```python
from build123d import *

# Parameters (mm, degrees)
SKETCH1_W           = 44.45
SKETCH1_H           = 25.4
BOSS_EXTRUDE1_DEPTH = 28.575
SHELL1_T            = -3.175
SKETCH2_W           = 38.1
SKETCH2_H           = 12.7
CUT_EXTRUDE1_DEPTH  = 26.4
CUT_EXTRUDE2_DEPTH  = 45.45
CUT_EXTRUDE3_DEPTH  = 4.175
FILLET1_R           = 6.35
FILLET2_R           = 1.5875
SKETCH6_R           = 9.525
CUT_EXTRUDE4_DEPTH  = 1.905


with BuildPart() as part:
    # Sketch1 → Boss-Extrude1 (new body)
    with BuildSketch(Plane(origin=(0, 0, 0), x_dir=(1, 0, 0), z_dir=(0, 1, 0))):
        with Locations((22.225, 12.7)):
            Rectangle(SKETCH1_W, SKETCH1_H)
    extrude(amount=BOSS_EXTRUDE1_DEPTH)

    # Shell1
    shell1_openings = [part.faces().sort_by_distance(p)[0] for p in [
        (22.225, 28.575, -12.7),
    ]]
    offset(amount=SHELL1_T, openings=shell1_openings, kind=Kind.INTERSECTION)

    # Sketch2 → Cut-Extrude1 (cut, through all)
    with BuildSketch(Plane.XY):
        with Locations((22.225, 22.225)):
            Rectangle(SKETCH2_W, SKETCH2_H)
    extrude(amount=-CUT_EXTRUDE1_DEPTH, mode=Mode.SUBTRACT)

    # Sketch3 → Cut-Extrude2 (cut, through all)
    with BuildSketch(Plane.ZY):
        with BuildLine():
            Line((-10.414, 23.8125), (-10.414, 20.6375))
            ThreePointArc((-10.414, 20.6375), (-12.7, 18.3515), (-14.986, 20.6375))
            Line((-14.986, 20.6375), (-14.986, 23.8125))
            ThreePointArc((-14.986, 23.8125), (-12.7, 26.0985), (-10.414, 23.8125))
        make_face()
    extrude(amount=-CUT_EXTRUDE2_DEPTH, mode=Mode.SUBTRACT)

    # Sketch5 → Cut-Extrude3 (cut, through all)
    with BuildSketch(Plane(origin=(0, 3.175, 0), x_dir=(1, 0, 0), z_dir=(0, 1, 0))):
        with BuildLine():
            Line((25.199729326, 6.5913), (19.250270674, 6.5913))
            ThreePointArc((19.250270674, 6.5913), (22.225, 19.4945), (25.199729326, 6.5913))
        make_face()
    extrude(amount=-CUT_EXTRUDE3_DEPTH, mode=Mode.SUBTRACT)

    # Fillet1
    fillet1_edges = [part.edges().sort_by_distance(p)[0] for p in [
        (42.8625, 28.575, -25.4),
        (1.5875, 28.575, -25.4),
        (42.8625, 28.575, 0),
        (1.5875, 28.575, 0),
    ]]
    fillet(fillet1_edges, radius=FILLET1_R)

    # Fillet2
    fillet2_edges = [part.edges().sort_by_distance(p)[0] for p in [
        (44.45, 26.715128061, -1.859871939),
        (44.45, 26.715128061, -23.540128061),
        (22.225, 0, -25.4),
        (44.45, 0, -12.7),
        (22.225, 0, 0),
        (0, 0, -12.7),
        (0, 28.575, -12.7),
        (0, 11.1125, 0),
        (0, 11.1125, -25.4),
        (0, 26.715128061, -1.859871939),
        (0, 26.715128061, -23.540128061),
        (44.45, 11.1125, -25.4),
        (44.45, 11.1125, 0),
        (44.45, 28.575, -12.7),
    ]]
    fillet(fillet2_edges, radius=FILLET2_R)

    # Sketch6 → Cut-Extrude4 (cut)
    with BuildSketch(Plane(origin=(0, 3.175, 0), x_dir=(1, 0, 0), z_dir=(0, 1, 0))):
        with Locations((22.225, 12.7)):
            Circle(SKETCH6_R)
    extrude(amount=-CUT_EXTRUDE4_DEPTH, mode=Mode.SUBTRACT)


solid = part.part
```
Source: CAD feature listing. Evaluate the final solid. Frame: model axes, mm. A direction names the side the tool comes from. Give positions to 0.01 mm unless a question says otherwise; leave off trailing zeros. Order: outer loops, then holes, each group sorted by start corner. A loop starts at its lowest first (then second) coordinate and runs counter-clockwise, first axis right, second up. Notation, with made-up numbers: (58.5, -8.75) -> (114.5, -8.75) arc R25 ccw to (114.5, 11.25) -> close; hole circle Ø8 at (-12.5, 74). An arc over 180 degrees is marked (long way). Use a Markdown table: item, result.
Q1. Section B-B (z = -12.7). State how many separate pieces and enclosed holes the cut face has, and give its area (3 significant figures).
A:
| item | result |
|---|---|
| separate pieces | 4 |
| enclosed holes | 0 |
| area | 198 mm^2 |
Q2. Section D-D (x = 7). Return the cut outline in (y, z) (1 decimal), and give its area (3 significant figures).
A:
| item | result |
|---|---|
| outline | (0, -23.8) arc R1.6 ccw to (1.6, -25.4) -> (15.9, -25.4) -> (15.9, -22.2) -> (3.2, -22.2) -> (3.2, -3.2) -> (15.9, -3.2) -> (15.9, 0) -> (1.6, 0) arc R1.6 ccw to (0, -1.6) -> close |
| area | 160 mm^2 |
Q3. Access query for faces 4 (the face through (43, 22, -14.986)), 5 (the face through (22, 9, -22.225)), 6 (the face through (22, 1, -6.591)). Directions: +Z, -Z, +X, -X, +Y, -Y. A direction counts if a zero-diameter tool reaches every point of the face in a straight line with its end or side. Return the directions, or none.
A:
| item | result |
|---|---|
| face 4 | +X, -X |
| face 5 | +Y |
| face 6 | +Y, -Y |
Q4. Pull-direction query (X, two-part tool) for faces 1 (the face through (3.175, 16, -13)), 2 (the face through (43.997, 28.098, -12.789)), 3 (the face through (2, 22, -10.414)); classes: +X half, -X half, draft (parallel to the pull), parting line (faces both ways), or undercut.
A:
| item | result |
|---|---|
| face 1 | undercut |
| face 2 | +X half |
| face 3 | draft |
Q5. Material intervals for line 1 (X direction, y = 2.1, z = -12.7); line 2 (X direction, y = 5.75, z = -21.75) (3 decimals); line 3 (Z direction, x = 30, y = 8.75) (3 decimals), sorted ascending. Write a range as [from, to].
A:
| item | result |
|---|---|
| line 1 | [0, 12.7], [31.75, 44.45] |
| line 2 | [0, 3.175], [41.275, 44.45] |
| line 3 | [-25.4, -22.225], [-3.175, 0] |
Q6. First-contact query: P1, Ø2.5, axis at x = 20, z = -2, coming from the +Y side (3 decimals); P2, Ø1, axis at x = 21, y = 1, coming from the -Z side; P3, Ø15, axis at x = 22.225, z = -12.7, coming from the +Y side. Flat tips, straight axial feed; report the tip coordinate or a pass-through.
A:
| item | result |
|---|---|
| P1 | y = 15.875 |
| P2 | z = -25.4 |
| P3 | y = 1.27 |
